Design review of the part built by this model. Coordinates are the model's own, in mm. A direction names the side the tool comes from. Give positions to 0.01 mm unless a question says otherwise; leave off trailing zeros. Write each loop counter-clockwise with the first axis right and the second up, starting at its lowest first coordinate (ties: lowest second). Pieces come first, ordered by that corner, then holes. Notation, with made-up numbers: (-25.5, 3.25) -> (6.5, 3.25) arc R34 ccw to (6.5, 36.25) -> close; hole circle Ø9 at (-26.5, 77). An arc over 180 degrees is marked (long way). Put each result on its own line as item: value. Start each with the question number.
from build123d import *

# Parameters (mm, degrees)
F0_W     = 40
F0_H     = 40
F1_DEPTH = 40
F2_T     = -4.5
F3_SIZE  = 35.5


with BuildPart() as f1:
    # F0 (on Top) → F1 (new body)
    with BuildSketch(Plane.XY):
        Rectangle(F0_W, F0_H)
    extrude(amount=F1_DEPTH)

    # F2
    f2_openings = [f1.faces().sort_by_distance(p)[0] for p in [
        (0, -20, 20),
        (0, 0, 40),
    ]]
    offset(amount=F2_T, openings=f2_openings)

    # F3
    f3_edges = [f1.edges().sort_by_distance(p)[0] for p in [
        (-17.75, -20, 40),
        (17.75, -20, 40),
    ]]
    chamfer(f3_edges, length=F3_SIZE)


solid = f1.part
Q1. Take a section at A-A on z = 36. Give the boundary of the cut face in (x, y), then the cut area to 3 significant figures.
Q2. Mouldability with a two-part tool opening along X and no side actions: class faces 3 (the face through (-17.8, -2, 22.5)), 4 (the face through (0, -2, 4.5)), 5 (the face through (20, 4, 15)) as +X half, -X half, draft (parallel to the pull), parting line (faces both ways), or undercut.
Q3. Take a section at C-C on x = -17. Give the boundary of the cut face in (y, z), then the cut area to 3 significant figures.
Q4. Machinability: for faces 1 (the face through (0, 18, 40)), 2 (the face through (0, 15.5, 22)), which of the approach directions +Z, -Z, +X, -X, +Y, -Y give a long, thin tool a straight path to every point of the face, cutting with its end or side? Answer none if there is none.
Q5. Take a section at D-D on x = 6.5. Give the boundary of the cut face in (y, z).
Q6. For pin 1 (9.5 mm diameter, centred on x = -1, z = 16.5, fed in from -Y); pin 2 (1 mm diameter, centred on x = 2, y = -7, fed in from +Z); pin 3 (4 mm diameter, centred on y = -13.5, z = 12.5, fed in from -X), all flat-tipped, find the tip position at first contact; note any pin that passes through.
Q7. Take a section at B-B on y = 6.5. Give the boundary of the cut face in (x, z), then the cut area to 4 significant figures.
Q8. To check wall thickness, follow probe 1 along X at (y, z) = (-3, 11); probe 2 along Y at (x, z) = (-14.5, 35.5); probe 3 along Z at (x, y) = (-4.5, -14). State the ranges of each line that lie inside material, in increasing order. Write a range as from..to.
Result:
1. outline: (-20, 11.5) -> (-15.5, 11.5) -> (-15.5, 15.5) -> (15.5, 15.5) -> (15.5, 11.5) -> (20, 11.5) -> (20, 20) -> (-20, 20) -> close
1. area: 216 mm^2
2. face 3: draft
2. face 4: undercut
2. face 5: +X half
3. outline: (-20, 0) -> (20, 0) -> (20, 40) -> (15.5, 40) -> (-20, 4.5) -> close
3. area: 970 mm^2
4. face 1: +Z, +X, -X, +Y, -Y
4. face 2: +Z, -Y
5. outline: (-20, 0) -> (20, 0) -> (20, 40) -> (15.5, 40) -> (15.5, 4.5) -> (-20, 4.5) -> close
6. pin 1: stops at y = 15.5
6. pin 2: stops at z = 4.5
6. pin 3: stops at x = -20
7. outline: (-20, 0) -> (20, 0) -> (20, 31) -> (15.5, 31) -> (15.5, 4.5) -> (-15.5, 4.5) -> (-15.5, 31) -> (-20, 31) -> close
7. area: 418.5 mm^2
8. probe 1: x = -20..-15.5, 15.5..20
8. probe 2: y = 15.5..20
8. probe 3: z = 0..4.5
